CAD build for the part. Positions are in the model's coordinates, mm. Face numbers are marked on the shaded views. A direction names the side the tool comes from. Give positions to 0.01 mm unless a question says otherwise; leave off trailing zeros. Write each loop counter-clockwise with the first axis right and the second up, starting at its lowest first coordinate (ties: lowest second). Pieces come first, ordered by that corner, then holes. Notation, with made-up numbers: M 9,-20 L 40,-20 A22 ccw 40,-13 Z; hole C 51,17 d4. An arc over 180 degrees is marked long. One line per question, with ' | ' between items. Start each with the question number.
1. Pull direction Z, two halves, no side cores. Call the marked faces 1, 2 and 3: released by +Z, released by -Z, zero draft, split by the parting line, or undercut.
2. Cut at C-C, the plane z = -38. Write the cut outline in (x, y), then the cut area to 3 significant figures.
3. Cut at D-D, the plane x = 26. Write the cut outline in (y, z), then the cut area to 3 significant figures.
4. Cut at A-A, the plane z = -31. Write the cut outline in (x, y), then the cut area to 3 significant figures.
5. Which spindle directions (+Z, -Z, +X, -X, +Y, -Y) get a long thin tool onto all of the face, cutting with end or side? Do the marked faces 4, 5 and 6. Say none if no direction does.
6. Cut at B-B, the plane y = 13.75. Write the cut outline in (x, z), then the cut area to 3 significant figures.
7. Wall check: L1, parallel to X at y = 14, z = -31; L2, parallel to Y at x = 67, z = -50; L3, parallel to Z at x = 91, y = 24.25. Give the ranges that are in metal, low to high.
8. Flat gauge pins, fed straight in: pin 1 (1.5 mm diameter, centred on x = 61.5, z = -12.5, fed in from -Y); pin 2 (7.5 mm diameter, centred on x = 85, y = 13.5, fed in from -Z); pin 3 (2 mm diameter, centred on x = 83, y = 18.5, fed in from +Z); pin 4 (2 mm diameter, centred on y = 2.5, z = -54, fed in from -X). Where does each tip first touch, or does it go through?
Autodesk Inventor part; units mm, degrees
ref_plane "YZ Plane" through (0, 0, 0) normal (1, 0, 0) x (0, 1, 0)
ref_plane "XZ Plane" through (0, 0, 0) normal (0, 1, 0) x (-1, 0, 0)
ref_plane "XY Plane" through (0, 0, 0) normal (0, 0, 1) x (1, 0, 0)
sketch "Sketch1" plane through (0, 0, 0) normal (0, 1, 0) x (-1, 0, 0)
  line L0 (0, 0) -> (-99, 0)
  line L1 (-99, 0) -> (-99, -60)
  line L2 (-99, -60) -> (0, -60)
  line L3 (0, -60) -> (0, 0)
  line L4 (-83, -52) -> (-90, -52)
  line L5 (-90, -52) -> (-90, -8)
  line L6 (-90, -8) -> (-83, -8)
  line L7 (-83, -8) -> (-83, -52)
  dimension "d0" = 99
  dimension "d1" = 60
  dimension "d2" = 7
  dimension "d3" = 44
  dimension "d4" = 8
  dimension "d5" = 9
extrude "Extrusion1" add sketch "Sketch1" along normal blind 4
sketch "Sketch2" plane through (0, 4, 0) normal (0, 1, 0) x (1, 0, 0)
  line L0 (83, 8) -> (83, 52)
  line L1 (83, 52) -> (90, 52)
  line L2 (90, 52) -> (90, 8)
  line L3 (90, 8) -> (83, 8)
  line L4 (91.5, 53.5) -> (81.5, 53.5)
  line L5 (81.5, 53.5) -> (81.5, 6.5)
  line L6 (81.5, 6.5) -> (91.5, 6.5)
  line L7 (91.5, 6.5) -> (91.5, 53.5)
  point P0 (0, 0)
  dimension "d8" = 1.5
extrude "Extrusion2" add sketch "Sketch2" along normal blind 22
sketch "Sketch3" plane through (0, 4, 0) normal (0, 1, 0) x (1, 0, 0)
  line L0 (99, 60) -> (0, 60) construction
  line L1 (0, 60) -> (0, 0) construction
  line L2 (0, 0) -> (99, 0) construction
  line L3 (99, 0) -> (99, 60) construction
  line L4 (4, 56) -> (95, 56) construction
  line L5 (95, 56) -> (95, 4) construction
  line L6 (95, 4) -> (4, 4) construction
  line L7 (4, 4) -> (4, 56) construction
  line L8 (0, 30) -> (99, 30) construction
  line L9 (49.5, 0) -> (49.5, 60) construction
  line L10 (0, 50) -> (0, 60)
  line L11 (0, 60) -> (13.5, 60)
  line L12 (13.5, 60) -> (13.5, 56)
  line L13 (13.5, 56) -> (4, 56)
  line L14 (4, 56) -> (4, 50)
  line L15 (4, 50) -> (0, 50)
  line L16 (0, 34) -> (4, 34)
  line L17 (4, 34) -> (4, 42)
  line L18 (4, 42) -> (0, 42)
  line L19 (0, 42) -> (0, 34)
  line L20 (45.5, 56) -> (37.5, 56)
  line L21 (37.5, 56) -> (37.5, 60)
  line L22 (37.5, 60) -> (45.5, 60)
  line L23 (45.5, 60) -> (45.5, 56)
  line L24 (29.5, 56) -> (21.5, 56)
  line L25 (21.5, 56) -> (21.5, 60)
  line L26 (21.5, 60) -> (29.5, 60)
  line L27 (29.5, 60) -> (29.5, 56)
  line L28 (0, 10) -> (0, 0)
  line L29 (0, 0) -> (13.5, 0)
  line L30 (13.5, 0) -> (13.5, 4)
  line L31 (13.5, 4) -> (4, 4)
  line L32 (4, 4) -> (4, 10)
  line L33 (4, 10) -> (0, 10)
  line L34 (0, 26) -> (4, 26)
  line L35 (4, 26) -> (4, 18)
  line L36 (4, 18) -> (0, 18)
  line L37 (0, 18) -> (0, 26)
  line L38 (45.5, 4) -> (37.5, 4)
  line L39 (37.5, 4) -> (37.5, 0)
  line L40 (37.5, 0) -> (45.5, 0)
  line L41 (45.5, 0) -> (45.5, 4)
  line L42 (29.5, 4) -> (21.5, 4)
  line L43 (21.5, 4) -> (21.5, 0)
  line L44 (21.5, 0) -> (29.5, 0)
  line L45 (29.5, 0) -> (29.5, 4)
  line L46 (99, 60) -> (99, 0) construction
  line L47 (95, 4) -> (95, 56) construction
  line L48 (99, 50) -> (99, 60)
  line L49 (99, 60) -> (85.5, 60)
  line L50 (85.5, 60) -> (85.5, 56)
  line L51 (85.5, 56) -> (95, 56)
  line L52 (95, 56) -> (95, 50)
  line L53 (95, 50) -> (99, 50)
  line L54 (99, 34) -> (95, 34)
  line L55 (95, 34) -> (95, 42)
  line L56 (95, 42) -> (99, 42)
  line L57 (99, 42) -> (99, 34)
  line L58 (53.5, 56) -> (61.5, 56)
  line L59 (61.5, 56) -> (61.5, 60)
  line L60 (61.5, 60) -> (53.5, 60)
  line L61 (53.5, 60) -> (53.5, 56)
  line L62 (69.5, 56) -> (77.5, 56)
  line L63 (77.5, 56) -> (77.5, 60)
  line L64 (77.5, 60) -> (69.5, 60)
  line L65 (69.5, 60) -> (69.5, 56)
  line L66 (77.5, 4) -> (77.5, 0)
  line L67 (69.5, 4) -> (77.5, 4)
  line L68 (77.5, 0) -> (69.5, 0)
  line L69 (69.5, 0) -> (69.5, 4)
  line L70 (61.5, 4) -> (61.5, 0)
  line L71 (53.5, 0) -> (53.5, 4)
  line L72 (53.5, 4) -> (61.5, 4)
  line L73 (61.5, 0) -> (53.5, 0)
  line L74 (85.5, 0) -> (85.5, 4)
  line L75 (85.5, 4) -> (95, 4)
  line L76 (95, 4) -> (95, 10)
  line L77 (99, 0) -> (85.5, 0)
  line L78 (99, 10) -> (99, 0)
  line L79 (95, 10) -> (99, 10)
  line L80 (95, 18) -> (99, 18)
  line L81 (95, 26) -> (95, 18)
  line L82 (99, 18) -> (99, 26)
  line L83 (99, 26) -> (95, 26)
  dimension "d11" = 4
  dimension "d12" = 8
  dimension "d13" = 4
  dimension "d14" = 8
  dimension "d15" = 8
  dimension "d16" = 4
  dimension "d17" = 8
  dimension "d18" = 8
  dimension "d19" = 8
extrude "Extrusion3" cut sketch "Sketch3" against normal up to surface (4 mm away)
properties part number "top" material "PBT Plastic Black"
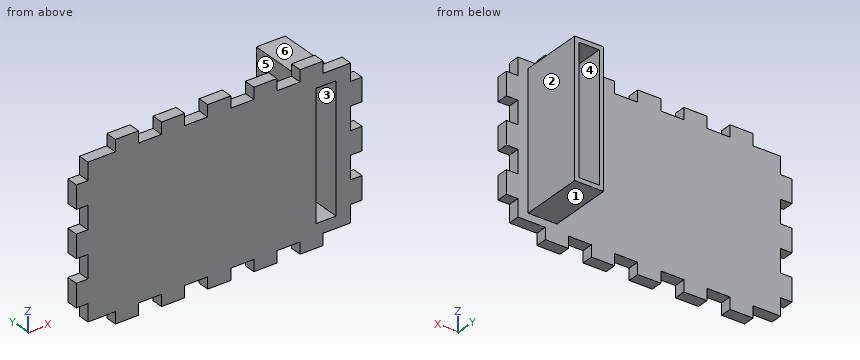
Here are the results:
1) face 1: released by -Z | face 2: zero draft | face 3: undercut
2) outline: M 4,0 L 83,0 L 83,26 L 81.5,26 L 81.5,4 L 4,4 Z; M 90,0 L 95,0 L 95,4 L 91.5,4 L 91.5,26 L 90,26 Z | area: 402 mm^2
3) outline: M 0,-56 L 4,-56 L 4,-4 L 0,-4 Z | area: 208 mm^2
4) outline: M 0,0 L 83,0 L 83,26 L 81.5,26 L 81.5,4 L 0,4 Z; M 90,0 L 99,0 L 99,4 L 91.5,4 L 91.5,26 L 90,26 Z | area: 434 mm^2
5) face 4: +Y, -Y | face 5: +Z, -Z, -X, +Y | face 6: +Z, +X, -X, +Y
6) outline: M 81.5,-53.5 L 91.5,-53.5 L 91.5,-6.5 L 81.5,-6.5 Z; hole M 83,-52 L 90,-52 L 90,-8 L 83,-8 Z | area: 162 mm^2
7) L1: 81.5 to 83, 90 to 91.5 | L2: 0 to 4 | L3: -53.5 to -6.5
8) pin 1: y = 0 | pin 2: z = -53.5 | pin 3: z = -6.5 | pin 4: x = 4
